Verification items for the finished model (mm, model axes). A direction names the side the tool comes from. Give positions to 0.01 mm unless a question says otherwise; leave off trailing zeros. Loops run counter-clockwise (first coordinate to the right, second up) from the corner with the lowest first, then second, coordinate; pieces in that order, holes last. Notation, with made-up numbers: (52.5, 69) - (68.5, 69) arc R17 cw to (68.5, 76) - close; hole circle Ø9 at (23, 39). An arc over 180 degrees is marked (long way). One line per question, with ' | ' between items. Start each with the question number.
1. Section check C-C, the plane z = 11. Enter the section's corners in (x, y) (3 decimals).
2. Mould release check, pull along X, two halves, no side actions. Record for faces 5 (the face through (20, -3.47, 39)), 6 (the face through (46.355, -11, 20)), 7 (the face through (23, 0, 20)): +X half, -X half, draft (parallel to the pull), parting line (faces both ways), or undercut.
3. Depth check by flat-ended pin: pin 1 Ø1.3 at (x, z) = (7.45, 17.57) entering from -Y; pin 2 Ø1 at (x, y) = (45.5, -11.5) entering from -Z; pin 3 Ø1 at (x, z) = (23, 39.5) entering from -Y; pin 4 Ø8 at (x, y) = (25, -19) entering from +Z. Enter the tip coordinate at first touch or a pass-through.
4. Thickness scan on line 1 along X through (y, z) = (-12.75, 12) (3 decimals); line 2 along Z through (x, y) = (42.5, -16.75) (3 decimals); line 3 along Y through (x, z) = (17, 35.5). Record the ranges inside material, lowest first. Write a range as from..to.
5. Section check A-A, the plane y = -13.75. Enter the section's corners in (x, z) (3 decimals), then the cut area to 3 significant figures.
6. Section check B-B, the plane x = 41.5. Enter the section's corners in (y, z) (3 decimals).
7. Section check D-D, the plane z = 30. Enter the section's corners in (x, y) (3 decimals), then the cut area to 3 significant figures.
8. Tool access check on faces 1 (the face through (36.43, -0.64, 17.85)), 2 (the face through (46, -12, 27.341)), 3 (the face through (28, -2, 38.735)), 4 (the face through (36.386, -13, 39)). Record the directions out of +Z, -Z, +X, -X, +Y, -Y that give a thin tool (end or side, any length) a straight path to the whole face; none if there is none.
from build123d import *

# Parameters (mm, degrees)
F0_W      = 46.355
F0_H      = 40.005
F1_DEPTH  = 21.59
F3_T      = -1.27
F5_W      = 26.924
F5_H      = 4.064
F6_DEPTH  = 63.246
F8_D      = 1.000001
F10_D     = 1.000001
F12_D     = 1.000001
F14_D     = 1.000001
F16_D     = 1.000001
F18_W     = 31.528105
F18_H     = 18.119926
F19_DEPTH = 25.4
F20_D     = 1.000001


with BuildPart() as f1:
    # F0 (on Front) → F1 (new body)
    with BuildSketch(Plane.XZ):
        with Locations((23.1775, 20.0025)):
            Rectangle(F0_W, F0_H)
    extrude(amount=F1_DEPTH)

    # F3
    f3_openings = [f1.faces().sort_by_distance(p)[0] for p in [
        (23.1775, -21.59, 20.0025),
    ]]
    offset(amount=F3_T, openings=f3_openings)

    # F5 (on Right) → F6 (cut)
    with BuildSketch(Plane.YZ):
        with Locations((-14.732, 29.373137)):
            Rectangle(F5_W, F5_H)
    extrude(amount=F6_DEPTH, mode=Mode.SUBTRACT)

    # F8 (through all)
    with Locations(Plane(origin=(0, 0, 0), x_dir=(-1, 0, 0), z_dir=(0, 1, 0))):
        with Locations((-10.5918, 17.609857)):
            Hole(F8_D / 2)

    # F10 (through all)
    with Locations(Plane(origin=(0, 0, 0), x_dir=(-1, 0, 0), z_dir=(0, 1, 0))):
        with Locations((-30.8102, 17.490488)):
            Hole(F10_D / 2)

    # F12 (through all)
    with Locations(Plane(origin=(0, 0, 0), x_dir=(-1, 0, 0), z_dir=(0, 1, 0))):
        with Locations((-33.4852, 17.490488)):
            Hole(F12_D / 2)

    # F14 (through all)
    with Locations(Plane(origin=(0, 0, 0), x_dir=(-1, 0, 0), z_dir=(0, 1, 0))):
        with Locations((-36.159544, 17.431264)):
            Hole(F14_D / 2)

    # F16 (through all)
    with Locations(Plane(origin=(0, 0, 0), x_dir=(-1, 0, 0), z_dir=(0, 1, 0))):
        with Locations((-7.450511, 17.565635)):
            Hole(F16_D / 2)

    # F18 (on face) → F19 (cut)
    with BuildSketch(Plane.XY.offset(40.005)):
        with Locations((20.622158, -12.530037)):
            Rectangle(F18_W, F18_H)
    extrude(amount=-F19_DEPTH, mode=Mode.SUBTRACT)

    # F20 (through all)
    with Locations(Plane(origin=(0, 0, 0), x_dir=(-1, 0, 0), z_dir=(0, 1, 0))):
        with Locations((-4.776387, 17.497179)):
            Hole(F20_D / 2)


solid = f1.part
Results list:
1) outline: (0, -21.59) - (1.27, -21.59) - (1.27, -1.27) - (45.085, -1.27) - (45.085, -21.59) - (46.355, -21.59) - (46.355, 0) - (0, 0) - close
2) face 5: undercut | face 6: +X half | face 7: draft
3) pin 1: y = -1.27 | pin 2: z = 0 | pin 3: y = -3.47 | pin 4: z = 1.27
4) line 1: 0..1.27, 45.085..46.355 | line 2: 0..1.27, 38.735..40.005 | line 3: -1.27..0
5) outline: (0, 0) - (46.355, 0) - (46.355, 27.341) - (45.085, 27.341) - (45.085, 1.27) - (1.27, 1.27) - (1.27, 27.341) - (0, 27.341) - close; (0, 31.405) - (1.27, 31.405) - (1.27, 38.735) - (4.858, 38.735) - (4.858, 40.005) - (0, 40.005) - close; (36.386, 38.735) - (45.085, 38.735) - (45.085, 31.405) - (46.355, 31.405) - (46.355, 40.005) - (36.386, 40.005) - close | area: 163 mm²
6) outline: (-21.59, 0) - (0, 0) - (0, 40.005) - (-21.59, 40.005) - (-21.59, 38.735) - (-1.27, 38.735) - (-1.27, 1.27) - (-21.59, 1.27) - close
7) outline: (0, -1.27) - (46.355, -1.27) - (46.355, 0) - (0, 0) - close | area: 58.9 mm²
8) face 1: +Y, -Y | face 2: +X, -X, -Y | face 3: -Y | face 4: +Z, -Y
